```python
from build123d import *

# Parameters (mm, degrees)
F0_R     = 7.5
F1_DEPTH = 52.80856
F2_R     = 57.7679652565
F2_R_2   = 7.5
F3_DEPTH = 3
F4_R     = 22.1047770768
F5_DEPTH = 84.87969
F6_R     = 18.757754514
F7_DEPTH = 25


with BuildPart() as f1:
    # F0 (on Front) → F1 (new body)
    with BuildSketch(Plane.XZ):
        with Locations((-53.8066774607, 33.8541828096)):
            Circle(F0_R)
    extrude(amount=F1_DEPTH)

    # F2 (on face) → F3 (join)
    with BuildSketch(Plane.XZ.offset(52.80856)):
        with Locations((-53.8066774607, 33.8541828096)):
            Circle(F2_R)
        with Locations((-53.8066774607, 33.8541828096)):
            Circle(F2_R_2, mode=Mode.SUBTRACT)
        with Locations((-53.8066774607, 33.8541828096)):
            Circle(F2_R)
    extrude(amount=F3_DEPTH)

    # F4 (on face) → F5 (join)
    with BuildSketch(Plane.XZ.offset(55.80856)):
        with Locations((-53.8066774607, 33.8541828096)):
            Circle(F4_R)
    extrude(amount=F5_DEPTH)

    # F6 (on face) → F7 (cut)
    with BuildSketch(Plane.XZ.offset(140.68825)):
        with Locations((-53.8066774607, 33.8541828096)):
            Circle(F6_R)
    extrude(amount=-F7_DEPTH, mode=Mode.SUBTRACT)


solid = f1.part
```
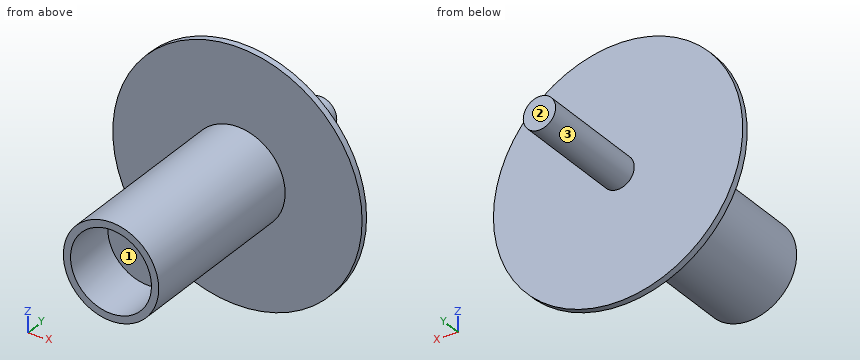
The listing builds one solid part. Answer for the finished solid, in the listing's coordinates (mm). Face numbers are marked on the shaded views. Give positions to 0.01 mm unless a question says otherwise; leave off trailing zeros. Write each loop counter-clockwise with the first axis right and the second up, starting at its lowest first coordinate (ties: lowest second). Pieces come first, ordered by that corner, then holes. Notation, with made-up numbers: (-35, 29) -> (9, 29) arc R25 cw to (9, 41) -> close; hole circle Ø9 at (46, 11). An arc over 180 degrees is marked (long way). Use one line per item in the form item = value.
1) Section B-B on x = -39 is taken. Write down the section's boundary in (y, z).
Result:
outline = (-140.69, 17.44) -> (-55.81, 17.44) -> (-55.81, -21.98) -> (-52.81, -21.98) -> (-52.81, 89.69) -> (-55.81, 89.69) -> (-55.81, 50.27) -> (-140.69, 50.27) -> (-140.69, 45.37) -> (-115.69, 45.37) -> (-115.69, 22.34) -> (-140.69, 22.34) -> close
2) For a pull along X with two mould halves and no side action, classify the marked faces 1, 2 and 3 as +X half, -X half, draft (parallel to the pull), parting line (faces both ways), or undercut.
Result:
face_1 = undercut
face_2 = draft
face_3 = parting line
3) Each of these flat-tipped pins is pushed along its axis until it touches: P1, Ø19, axis at x = -55.5, z = 31, coming from the -Y side; P2, Ø4, axis at y = -114, z = 24.5, coming from the +X side; P3, Ø6, axis at x = -35.5, z = 30.5, coming from the +Y side. Where does it stop, or does it pass through?
Result:
P1 = -115.69
P2 = -32.96
P3 = -52.81
4) Section D-D on z = 79.5 is taken. Write down the section's boundary in (x, y).
Result:
outline = (-89.21, -55.81) -> (-18.4, -55.81) -> (-18.4, -52.81) -> (-89.21, -52.81) -> close
5) Section C-C on y = -62 is taken. Write down the section's boundary in (x, z).
Result:
outline = circle Ø44.21 at (-53.81, 33.85)
6) Section A-A on z = 23 is taken. Write down the section's boundary in (x, y), plus the area to 3 significant figures.
Result:
outline = (-110.55, -55.81) -> (-73.06, -55.81) -> (-73.06, -140.69) -> (-69.11, -140.69) -> (-69.11, -115.69) -> (-38.51, -115.69) -> (-38.51, -140.69) -> (-34.55, -140.69) -> (-34.55, -55.81) -> (2.93, -55.81) -> (2.93, -52.81) -> (-110.55, -52.81) -> close
area = 2,840 mm²
7) Straight lines are drawn through the part: probe 1 along Z at (x, y) = (-53, -116); probe 2 along Z at (x, y) = (-63, -123); probe 3 along Y at (x, z) = (-69.5, 55). For each, find the intervals that lie inside material, in ascending order.
Result:
probe_1 = 11.76 to 15.11, 52.59 to 55.94
probe_2 = 13.75 to 17.5, 50.2 to 53.96
probe_3 = -55.81 to -52.81
